```python
from build123d import *

# Parameters (mm, degrees)
SKETCH1_W           = 25.4
SKETCH1_H           = 25.4
SKETCH1_W_2         = 19.05
SKETCH1_H_2         = 19.05
BOSS_EXTRUDE1_DEPTH = 101.6
SKETCH2_RX          = 3.175
SKETCH2_RY          = 3.173642052
CUT_EXTRUDE1_DEPTH  = 101.6


with BuildPart() as part:
    # Sketch1 → Boss-Extrude1 (new body)
    with BuildSketch(Plane.XY):
        with Locations((12.7, 12.7)):
            Rectangle(SKETCH1_W, SKETCH1_H)
        with Locations((12.7, 12.7)):
            Rectangle(SKETCH1_W_2, SKETCH1_H_2, mode=Mode.SUBTRACT)
    extrude(amount=BOSS_EXTRUDE1_DEPTH)

    # Sketch2 → Cut-Extrude1 (cut)
    with BuildSketch(Plane(origin=(0, 25.4, 0), x_dir=(1, 0, 0), z_dir=(0, 1, 0))):
        with Locations(Location((13.766367438, -53.764427429), (0, 0, -36.863751169))):
            Ellipse(SKETCH2_RX, SKETCH2_RY)
    extrude(amount=-CUT_EXTRUDE1_DEPTH, mode=Mode.SUBTRACT)


solid = part.part
```
The model under review builds one solid part; all positions refer to its coordinate system, in mm. A direction names the side the tool comes from. Give positions to 0.01 mm unless a question says otherwise; leave off trailing zeros. Write each loop counter-clockwise with the first axis right and the second up, starting at its lowest first coordinate (ties: lowest second). Pieces come first, ordered by that corner, then holes. Notation, with made-up numbers: (-3, 88.25) -> (44, 88.25) arc R16 ccw to (44, 103.25) -> close; hole circle Ø4 at (-36.5, 53.25). An arc over 180 degrees is marked (long way). Answer in a Markdown table with one row per item.
1) For L1, parallel to Y at x = 19, z = 14 (3 decimals), list the stretches that pass through material, from the lowest coordinate up. Write a range as [from, to].
Worked answers:
| item | result |
|---|---|
| L1 | [0, 3.175], [22.225, 25.4] |
2) Add section D-D on x = 14.5. Count the separate pieces of the cut face and the enclosed holes in it, plus the area to 3 significant figures.
Worked answers:
| item | result |
|---|---|
| separate pieces | 4 |
| enclosed holes | 0 |
| area | 606 mm² |
3) Mouldability with a two-part tool opening along X and no side actions: class faces 1 (the flat face through (22.225, 13, 50)), 2 (the flat face through (25.4, 13, 50)), 3 (the flat face through (24, 13, 0)) as +X half, -X half, draft (parallel to the pull), parting line (faces both ways), or undercut.
Worked answers:
| item | result |
|---|---|
| face 1 | undercut |
| face 2 | +X half |
| face 3 | draft |
4) Add section A-A on x = 19.25. State the section outline as (y, z) points (3 decimals).
Worked answers:
| item | result |
|---|---|
| outline | (0, 0) -> (3.175, 0) -> (3.175, 101.6) -> (0, 101.6) -> close; (22.225, 0) -> (25.4, 0) -> (25.4, 101.6) -> (22.225, 101.6) -> close |
5) Tool access review of faces 4 (the flat face through (13, 0, 50)), 5 (the flat face through (13, 22.225, 50)): name each direction out of +Z, -Z, +X, -X, +Y, -Y from which nothing blocks a thin tool from reaching the whole face with its end or side.
Worked answers:
| item | result |
|---|---|
| face 4 | +Z, -Z, +X, -X, -Y |
| face 5 | +Z, -Z |
6) Add section C-C on z = 94.5. State the section outline as (x, y) points (3 decimals), plus the area to 3 significant figures.
Worked answers:
| item | result |
|---|---|
| outline | (0, 0) -> (25.4, 0) -> (25.4, 25.4) -> (0, 25.4) -> close; hole (3.175, 3.175) -> (22.225, 3.175) -> (22.225, 22.225) -> (3.175, 22.225) -> close |
| area | 282 mm² |
